Input: dimensioned drawing with shaded views. Units: mm. Origin: part minimum x, y, z. Round coordinates to 2 decimals unless told otherwise and drop trailing zeros. Order: outer loops, then holes, each group sorted by start corner. A loop starts at its lowest first (then second) coordinate and runs counter-clockwise, first axis right, second up. Notation, with made-up numbers: (-26.5, -8) - (9.5, -8) arc R27 cw to (9.5, 16) - close; hole circle Ø6 at (24.5, 11). An arc over 180 degrees is marked (long way). Put each result on its own line as item: value. Start each with the question number.
(1) Pin query (flat end, axial travel): P1, Ø4, axis at x = 86.5, y = 8.5, coming from the +Z side; P2, Ø10, axis at x = 119, z = 99, coming from the +Y side (1 decimal); P3, Ø8, axis at x = 110.5, y = 4.5, coming from the +Z side. Return the tip coordinate at first contact, or that it passes through.
(2) Section C-C (x = 29.5). Output: boundary loops of the cut face in (y, z), and give its area (3 significant figures).
(3) Material intervals for L1, parallel to X at y = 11.75, z = 100; L2, parallel to Z at x = 109, y = 8.75 (1 decimal); L3, parallel to Z at x = 83.5, y = 10.75 (1 decimal), sorted ascending. Write a range as [from, to].
(4) Section A-A (z = 100). Output: boundary loops of the cut face in (x, y) (1 decimal).
(5) Section B-B (y = 10.25). Output: boundary loops of the cut face in (x, z), and give its area (3 significant figures).
(6) Section D-D (z = 28). Output: boundary loops of the cut face in (x, y), and give its area (3 significant figures).
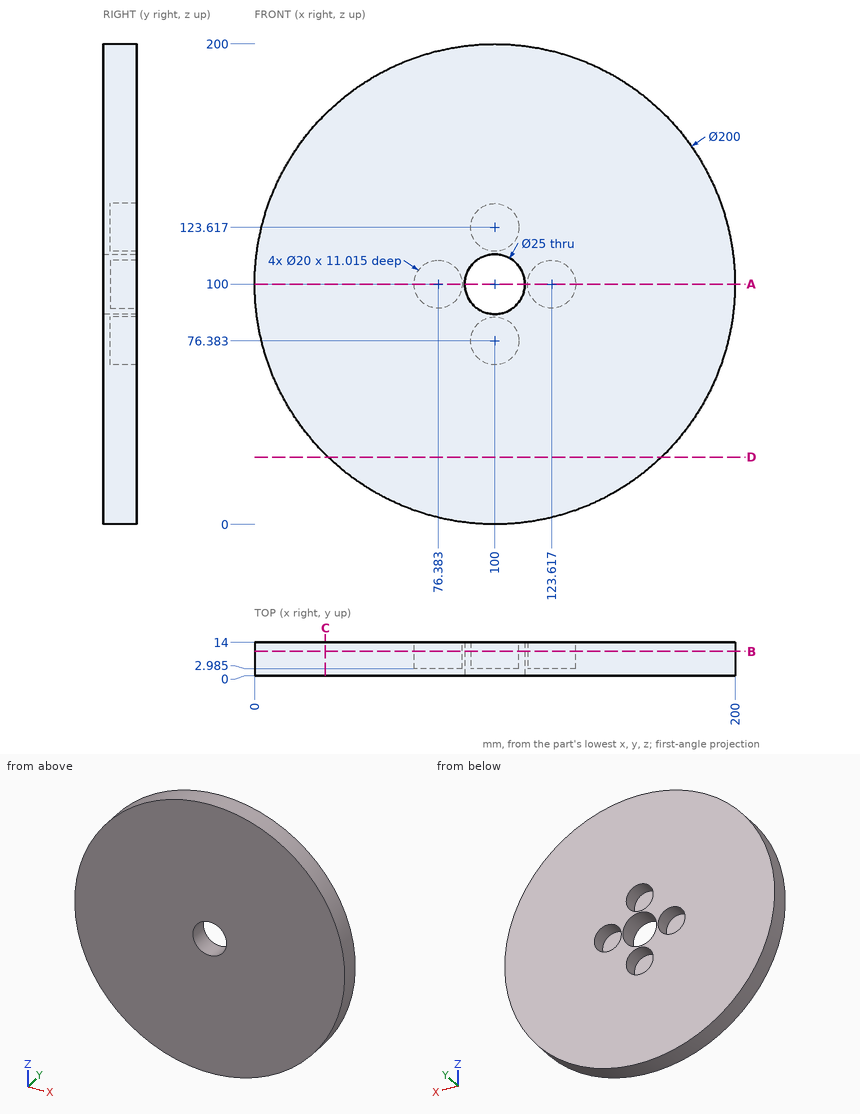
Checks:
1. P1: stops at z = 199.34
1. P2: stops at y = 3
1. P3: stops at z = 199.79
2. outline: (0, 29.08) - (14, 29.08) - (14, 170.92) - (0, 170.92) - close
2. area: 1,990 mm²
3. L1: x = [0, 66.38], [86.38, 87.5], [112.5, 113.62], [133.62, 200]
3. L2: z = [0.4, 72], [80.7, 91.3], [108.7, 119.3], [128, 199.6]
3. L3: z = [1.4, 93], [107, 198.6]
4. outline: (0, 0) - (87.5, 0) - (87.5, 14) - (86.4, 14) - (86.4, 3) - (66.4, 3) - (66.4, 14) - (0, 14) - close; (112.5, 0) - (200, 0) - (200, 14) - (133.6, 14) - (133.6, 3) - (113.6, 3) - (113.6, 14) - (112.5, 14) - close
5. outline: circle Ø200 at (100, 100); hole circle Ø20 at (76.38, 100); hole circle Ø25 at (100, 100); hole circle Ø20 at (100, 76.38); hole circle Ø20 at (100, 123.62); hole circle Ø20 at (123.62, 100)
5. area: 29,700 mm²
6. outline: (30.6, 0) - (169.4, 0) - (169.4, 14) - (30.6, 14) - close
6. area: 1,940 mm²
